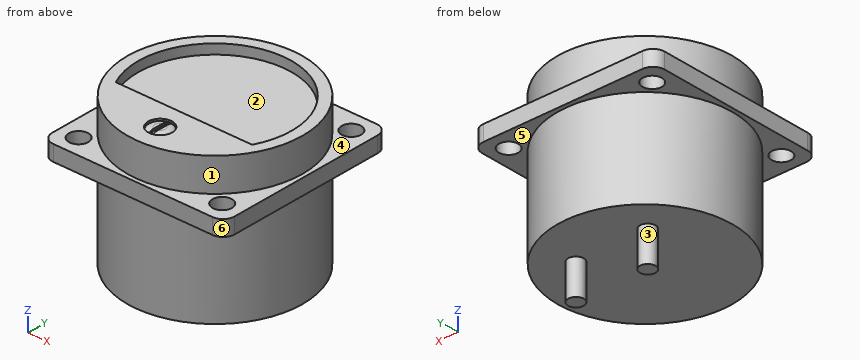
Autodesk Inventor part; units mm, degrees
ref_plane "YZ Plane" through (0, 0, 0) normal (1, 0, 0) x (0, 1, 0)
ref_plane "XZ Plane" through (0, 0, 0) normal (0, 1, 0) x (-1, 0, 0)
ref_plane "XY Plane" through (0, 0, 0) normal (0, 0, 1) x (1, 0, 0)
sketch "Base" plane through (0, 0, 0) normal (0, 0, 1) x (1, 0, 0)
  line L0 (-23.5, -23.5) -> (23.5, -23.5)
  line L1 (23.5, -23.5) -> (23.5, 23.5)
  line L2 (23.5, 23.5) -> (-23.5, 23.5)
  line L3 (-23.5, 23.5) -> (-23.5, -23.5)
  line L4 (-23.5, -23.5) -> (23.5, 23.5) construction
  line L5 (23.5, -23.5) -> (-23.5, 23.5) construction
  point P0 (0, 0)
  dimension "d0" = 47
extrude "BaseFeature" add sketch "Base" along normal blind 4
fillet "FilletsFeature" radius 3 4 edges at (-23.5, -23.5, 2) (-23.5, 23.5, 2) (23.5, -23.5, 2) (23.5, 23.5, 2)
sketch "Front" plane through (0, 0, 4) normal (0, 0, 1) x (1, 0, 0)
  circle A0 centre (0, 0) radius 22.5
  dimension "d4" = 45
extrude "FrontFeature" add sketch "Front" along normal blind 8.5
sketch "Screen" plane through (0, 0, 12.5) normal (0, 0, 1) x (1, 0, 0)
  circle A0 centre (0, 0) radius 19.7
  circle A1 centre (0, 0) radius 22.5
  line L0 (-17.575, -8.9) -> (17.575, -8.9)
  line L1 (0, -8.9) -> (0, -19.7) construction
  dimension "d7" = 2.8
  dimension "d8" = 10.8
extrude "ScreenFEature" cut sketch "Screen" against normal blind 2.5 contours A0 L0 picked at (4.7799, 0.8366)
sketch "ScrewHole" plane through (0, 0, 12.5) normal (0, 0, 1) x (1, 0, 0)
  line L0 (17.575, -8.9) -> (-17.575, -8.9)
  line L1 (0, -8.9) -> (0, -22.5) construction
  circle A0 centre (0, 0) radius 22.5
  circle A1 centre (0, -15.7) radius 3
  circle A2 centre (0, -15.7) radius 3.1
  dimension "d11" = 6
  dimension "d12" = 0.1
extrude "ScrewHoleFeature" cut sketch "ScrewHole" against normal blind 0.5 contours A1 | A2
sketch "ScrewHead" plane through (0, -15.7, 12) normal (0, 0, 1) x (1, 0, 0)
  circle A0 centre (0, 0) radius 3
  circle A1 centre (0, 0) radius 3.1
  point P0 (0, 15.7)
  dimension "d15" = 6
extrude "ScrewHeadFeature" add sketch "ScrewHead" along normal blind 0.5 contours A0
fillet "ScrewHeadFilletFeature" radius 3 1 edges at (-3, -15.7, 12.5)
sketch "ScrewFlat" plane through (0, -15.7, 12.5) normal (0, 0, 1) x (1, 0, 0)
  circle A0 centre (0, 0) radius 3
  line L0 (0, 3) -> (0, -3) construction
  line L1 (-0.5, -2.5) -> (0.5, -2.5)
  line L2 (0.5, -2.5) -> (0.5, 2.5)
  line L3 (0.5, 2.5) -> (-0.5, 2.5)
  line L4 (-0.5, 2.5) -> (-0.5, -2.5)
  circle A1 centre (0, 0) radius 1.3417
  line L5 (-0.5, -2.5) -> (0.5, 2.5) construction
  line L6 (0.5, -2.5) -> (-0.5, 2.5) construction
  point P0 (0, 15.7)
  dimension "d19" = 5
  dimension "d20" = 1
extrude "ScrewFlatFeature" cut sketch "ScrewFlat" against normal blind 0.5 contours L4 A1 L2 L1 | L4 A1 L2 | L4 L3 L2 A1
sketch "MountHoles" plane through (0, 0, 4) normal (0, 0, 1) x (1, 0, 0)
  circle A0 centre (-18.5, -18.5) radius 2.5
  line L0 (-32.9, 0) -> (32.9, 0)
  line L1 (0, -32.9) -> (0, 32.9)
  circle A1 centre (18.5, -18.5) radius 2.5
  circle A2 centre (-18.5, 18.5) radius 2.5
  circle A3 centre (18.5, 18.5) radius 2.5
  point P0 (0, 0)
  dimension "d23" = 5
  dimension "d24" = 37
  dimension "d25" = 37
extrude "MountHolesFeature" cut sketch "MountHoles" against normal through all
sketch "Body" plane through (0, 0, 0) normal (0, 0, -1) x (-1, 0, 0)
  circle A0 centre (0, 0) radius 22.5
extrude "BodyFeature" add sketch "Body" along normal blind 25
sketch "Studs" plane through (0, 0, -25) normal (0, 0, -1) x (-1, 0, 0)
  circle A0 centre (0, 0) radius 22.5
  line L0 (-21.2132, 7.5) -> (21.2132, 7.5) construction
  circle A1 centre (9.25, 9.5) radius 2
  line L1 (0, -32.9) -> (0, 32.9) construction
  circle A2 centre (-9.25, 9.5) radius 2
  line L2 (9.25, 9.5) -> (9.25, 7.5) construction
  line L3 (-9.25, 9.5) -> (-11.25, 9.5) construction
  line L4 (9.25, 9.5) -> (11.25, 9.5) construction
  point P0 (0, 22.5)
  dimension "d32" = 4
  dimension "d30" = 15
  dimension "d31" = 22.5
extrude "StudsFeature" add sketch "Studs" along normal blind 9 contours A1 | A2
equation "\"d25\" = d24"
properties part number "BaomanACPanelMountMeter"
Source: CAD feature listing. Evaluate the final solid. Frame: model axes, mm. Face numbers are marked on the shaded views. A direction names the side the tool comes from. Give positions to 0.01 mm unless a question says otherwise; leave off trailing zeros. Write each loop counter-clockwise with the first axis right and the second up, starting at its lowest first coordinate (ties: lowest second). Pieces come first, ordered by that corner, then holes. Notation, with made-up numbers: (40, -28) -> (87, -28) arc R22 ccw to (87, -5) -> close; hole circle Ø2 at (-21.75, 45.5). An arc over 180 degrees is marked (long way). Return JSON: item names as keys, results as strings. Group by question number.
1. Material intervals for line 1 (Y direction, x = 18.5, z = 1.15); line 2 (X direction, y = -18, z = 1); line 3 (Z direction, x = -18, y = -15.5), sorted ascending. Write a range as from..to.
2. Mould query, pull axis X, two halves, no side actions, for the marked faces 1, 2, 3 and 4. Classes: +X half, -X half, draft (parallel to the pull), parting line (faces both ways), or undercut.
3. Section C-C, the plane z = -29. Output: boundary loops of the cut face in (x, y).
4. Access query for the marked faces 5 and 6. Directions: +Z, -Z, +X, -X, +Y, -Y. A direction counts if a zero-diameter tool reaches every point of the face in a straight line with its end or side. Return the directions, or none.
5. Section B-B, the plane x = -10.5. Output: boundary loops of the cut face in (y, z), then the cut area to 3 significant figures.
6. Pin query (flat end, axial travel): pin 1 Ø7 at (x, y) = (0, -15.7) entering from +Z; pin 2 Ø0.8 at (x, z) = (7.5, 11) entering from +Y; pin 3 Ø2 at (x, y) = (7.5, -1.5) entering from +Z; pin 4 Ø4 at (y, z) = (-9.5, -25) entering from +X. Return the tip coordinate at first contact, or that it passes through.
7. Section D-D, the plane y = 12.5. Output: boundary loops of the cut face in (x, z).
8. Section A-A, the plane y = 18.5. Output: boundary loops of the cut face in (x, z).
Determined:
{
 "1": {"line 1": "y = -23.5..-21, -16..16, 21..23.5", "line 2": "x = -23.5..-20.95, -16.05..16.05, 20.95..23.5", "line 3": "z = 0..4"},
 "2": {"face 1": "parting line", "face 2": "undercut", "face 3": "undercut", "face 4": "draft"},
 "3": {"outline": "circle Ø4 at (-9.25, 9.5); circle Ø4 at (9.25, 9.5)"},
 "4": {"face 5": "-Z", "face 6": "+Z, -Z, +X, -Y"},
 "5": {"outline": "(-23.5, 0) -> (-19.9, 0) -> (-19.9, -25) -> (7.94, -25) -> (7.94, -34) -> (11.06, -34) -> (11.06, -25) -> (19.9, -25) -> (19.9, 0) -> (23.5, 0) -> (23.5, 4) -> (19.9, 4) -> (19.9, 12.5) -> (16.67, 12.5) -> (16.67, 10) -> (-8.9, 10) -> (-8.9, 12.5) -> (-19.9, 12.5) -> (-19.9, 4) -> (-23.5, 4) -> close", "area": "1,490 mm2"},
 "6": {"pin 1": "stops at z = 12.5", "pin 2": "stops at y = 21.35", "pin 3": "stops at z = 10", "pin 4": "stops at x = 21.21"},
 "7": {"outline": "(-23.5, 0) -> (-18.71, 0) -> (-18.71, -25) -> (18.71, -25) -> (18.71, 0) -> (23.5, 0) -> (23.5, 4) -> (18.71, 4) -> (18.71, 12.5) -> (15.23, 12.5) -> (15.23, 10) -> (-15.23, 10) -> (-15.23, 12.5) -> (-18.71, 12.5) -> (-18.71, 4) -> (-23.5, 4) -> close"},
 "8": {"outline": "(-23.5, 0) -> (-21, 0) -> (-21, 4) -> (-23.5, 4) -> close; (-16, 0) -> (-12.81, 0) -> (-12.81, -25) -> (12.81, -25) -> (12.81, 0) -> (16, 0) -> (16, 4) -> (12.81, 4) -> (12.81, 12.5) -> (6.77, 12.5) -> (6.77, 10) -> (-6.77, 10) -> (-6.77, 12.5) -> (-12.81, 12.5) -> (-12.81, 4) -> (-16, 4) -> close; (21, 0) -> (23.5, 0) -> (23.5, 4) -> (21, 4) -> close"}
}
